Autodesk Inventor part; units mm, degrees
ref_plane "YZ Plane" through (0, 0, 0) normal (1, 0, 0) x (0, 1, 0)
ref_plane "XZ Plane" through (0, 0, 0) normal (0, 1, 0) x (-1, 0, 0)
ref_plane "XY Plane" through (0, 0, 0) normal (0, 0, 1) x (1, 0, 0)
sketch "Szkic1" plane through (0, 0, 0) normal (0, 1, 0) x (-1, 0, 0)
  line L0 (0, 0) -> (20, 0)
  line L1 (20, 0) -> (20, -25)
  line L2 (20, -25) -> (0, -25)
  line L3 (0, -25) -> (0, 0)
  line L4 (0, -25) -> (20, -25)
  line L5 (20, -25) -> (20, -30)
  line L6 (20, -30) -> (0, -30)
  line L7 (0, -30) -> (0, -25)
  line L8 (0, -30) -> (20, -30)
  line L9 (0, -30) -> (20, -30)
  line L10 (20, -30) -> (20, -55)
  line L11 (20, -55) -> (0, -55)
  line L12 (0, -55) -> (0, -30)
  line L13 (0, -55) -> (20, -55)
  line L14 (20, -55) -> (20, -60)
  line L15 (20, -60) -> (0, -60)
  line L16 (0, -60) -> (0, -55)
  line L17 (0, -60) -> (12.1994, -60)
  line L18 (0, -60) -> (20, -60)
  line L19 (20, -60) -> (20, -85)
  line L20 (20, -85) -> (0, -85)
  line L21 (0, -85) -> (0, -60)
  line L22 (0, -85) -> (20, -85)
  line L23 (20, -85) -> (20, -90)
  line L24 (20, -90) -> (0, -90)
  line L25 (0, -90) -> (0, -85)
  line L26 (0, -90) -> (12.1994, -90)
  line L27 (0, -90) -> (20, -90)
  line L28 (20, -90) -> (20, -115)
  line L29 (20, -115) -> (0, -115)
  line L30 (0, -115) -> (0, -90)
  line L31 (0, -115) -> (20, -115)
  line L32 (20, -115) -> (20, -120)
  line L33 (20, -120) -> (0, -120)
  line L34 (0, -120) -> (0, -115)
  line L35 (0, -120) -> (3.8166, -120)
  line L36 (20, -120) -> (0, -120)
  line L37 (0, -120) -> (0, -145)
  line L38 (0, -145) -> (20, -145)
  line L39 (20, -145) -> (20, -120)
  circle A0 centre (10, -7.5) radius 2.8
  circle A1 centre (10, -17.5) radius 2.8
  line L40 (20, -42.5) -> (0, -42.5) construction
  line L41 (20, -72.5) -> (0, -72.5) construction
  line L42 (20, -102.5) -> (0, -102.5) construction
  line L43 (20, -132.5) -> (0, -132.5) construction
  line L44 (20, -12.5) -> (0, -12.5) construction
  circle A2 centre (10, -47.5) radius 2.8
  circle A3 centre (10, -37.5) radius 2.8
  circle A4 centre (10, -77.5) radius 2.8
  circle A5 centre (10, -67.5) radius 2.8
  circle A6 centre (10, -107.5) radius 2.8
  circle A7 centre (10, -97.5) radius 2.8
  circle A8 centre (10, -137.5) radius 2.8
  circle A9 centre (10, -127.5) radius 2.8
  circle A10 centre (10, -167.5) radius 2.8
  circle A11 centre (10, -157.5) radius 2.8
  line L45 (20, -145) -> (0, -145)
  line L46 (0, -145) -> (0, -150)
  line L47 (0, -150) -> (20, -150)
  line L48 (20, -150) -> (20, -145)
  line L49 (20, -150) -> (0, -150)
  line L50 (0, -150) -> (0, -175)
  line L51 (0, -175) -> (20, -175)
  line L52 (20, -175) -> (20, -150)
  line L53 (20, -162.5) -> (0, -162.5) construction
  dimension "d2" = 20
  dimension "d3" = 25
  dimension "d4" = 5
  dimension "d14" = 10
  dimension "d16" = 10
  dimension "d17" = 5.6
  dimension "d20" = 30
extrude "Wyciągnięcie proste1" add sketch "Szkic1" along normal blind 4
extrude "Wyciągnięcie proste2" add sketch "Szkic1" against normal blind 5 contours L2 L5 L6 L7 | L11 L14 L15 L16 | L20 L23 L24 L25 | L29 L32 L33 L34 | L38 L48 L47 L46
fillet "Zaokrąglenie1" radius 1.6 24 edges at (0, 2, 0) (-20, 2, 0) (0, 2, -175) (-20, 2, -175) (-20, -2.5, -150) (0, -2.5, -150) (0, -2.5, -145) (-20, -2.5, -145) (0, -2.5, -120) (0, -2.5, -115) (-20, -2.5, -120) (-20, -2.5, -115) (-20, -2.5, -90) (-20, -2.5, -85) (0, -2.5, -90) (0, -2.5, -85) (0, -2.5, -60) (0, -2.5, -55) (-20, -2.5, -55) (-20, -2.5, -60) (-20, -2.5, -30) (-20, -2.5, -25) (0, -2.5, -25) (0, -2.5, -30)
equation "\"d16\" = 0.5 * d2"
properties part number "belka_poprzeg" material "PLA"
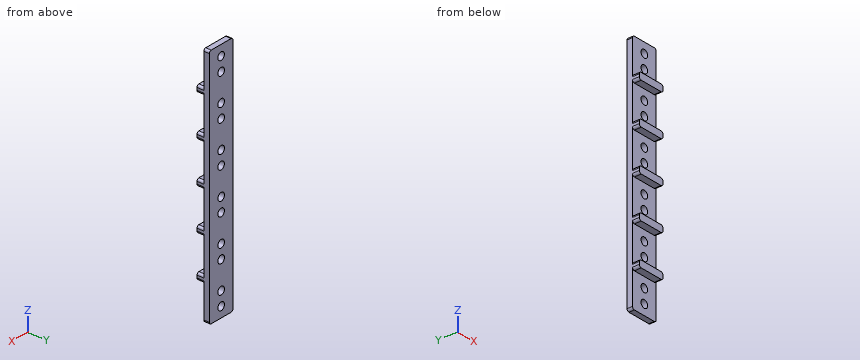
Can you work these out from the model? Positions are in its coordinate system, mm. Give positions to 0.01 mm unless a question says otherwise; leave off trailing zeros. Write each loop counter-clockwise with the first axis right and the second up, starting at its lowest first coordinate (ties: lowest second). Pieces come first, ordered by that corner, then holes. Notation, with made-up numbers: (-10.75, 13) -> (36.25, 13) arc R21 cw to (36.25, 24) -> close; hole circle Ø11 at (-9, -28). An arc over 180 degrees is marked (long way). Answer as a JSON object with one key per item and string values. Group by question number.
Item 1: I'm going to push flat-ended pins straight in: P1, Ø9, axis at x = -10, z = -37.5, coming from the -Y side; P2, Ø5, axis at x = -10, z = -167.5, coming from the -Y side; P3, Ø1.5, axis at x = -8, y = -2.5, coming from the -Z side; P4, Ø1.5, axis at x = -4.5, y = -1.5, coming from the +Z side. Where does each tip first touch, or does it pass through?
Item 2: Suppose I cut it at A-A (z = -127.5). Please give me the cut outline in (x, y).
Item 3: Please list where these lines run through material, in increasing order: line 1 (Z direction, x = -7.75, y = -2.25); line 2 (Y direction, x = -15.5, z = -19.5); line 3 (X direction, y = 1.5, z = -69.5). Write a range as [from, to].
Item 4: Suppose I cut it at B-B (y = 1.5). State how many separate pieces and enclosed holes the cut face has, plus the area to 3 significant figures.
Item 5: Suppose I cut it at C-C (x = -4.5). Please give me the cut outline in (y, z).
Findings:
{
 "1": {"P1": "stops at y = 0", "P2": "passes through", "P3": "stops at z = -150", "P4": "stops at z = -25"},
 "2": {"outline": "(-20, 0) -> (-12.8, 0) -> (-12.8, 4) -> (-20, 4) -> close; (-7.2, 0) -> (0, 0) -> (0, 4) -> (-7.2, 4) -> close"},
 "3": {"line 1": "z = [-150, -145], [-120, -115], [-90, -85], [-60, -55], [-30, -25]", "line 2": "y = [0, 4]", "line 3": "x = [-20, -11.96], [-8.04, 0]"},
 "4": {"separate pieces": "1", "enclosed holes": "12", "area": "3,200 mm²"},
 "5": {"outline": "(-5, -150) -> (0, -150) -> (0, -175) -> (4, -175) -> (4, 0) -> (0, 0) -> (0, -25) -> (-5, -25) -> (-5, -30) -> (0, -30) -> (0, -55) -> (-5, -55) -> (-5, -60) -> (0, -60) -> (0, -85) -> (-5, -85) -> (-5, -90) -> (0, -90) -> (0, -115) -> (-5, -115) -> (-5, -120) -> (0, -120) -> (0, -145) -> (-5, -145) -> close"}
}
